from build123d import *

# Parameters (mm, degrees)
F0_W     = 150
F0_H     = 75
F1_DEPTH = 4.8
F2_W     = 143
F2_H     = 1.4
F3_DEPTH = 2
F4_R     = 1.99999


# Not quite as in the source:
# - a fillet or chamfer is up to 0.001 mm smaller than in the source, because OpenCascade refuses the exact size


with BuildPart() as f1:
    # F0 (on Front) → F1 (new body)
    with BuildSketch(Plane.XZ):
        Rectangle(F0_W, F0_H)
    extrude(amount=F1_DEPTH)

    # F2 (on face) → F3 (cut)
    with BuildSketch(Plane.XZ.offset(4.8)):
        Polygon((68, 12.5), (68, -37.5), (73, -37.5), (73, 37.5), (68, 37.5), (68, 13.9), align=None)
        with Locations((-3.5, 13.2)):
            Rectangle(F2_W, F2_H)
    extrude(amount=-F3_DEPTH, mode=Mode.SUBTRACT)

    # F4 (radius 2 in the source; OpenCascade refuses exactly that, so slightly less here)
    f4_edges = [f1.edges().sort_by_distance(p)[0] for p in [
        (75, 0, 0),
        (75, -4.8, 0),
    ]]
    fillet(f4_edges, radius=F4_R)


solid = f1.part
Geometry: final body of the model. Coordinates: model frame, mm. Coordinates: 2 decimals unless noted, no trailing zeros. Order: outer loops, then holes, each group sorted by start corner. A loop starts at its lowest first (then second) coordinate and runs counter-clockwise, first axis right, second up.
(1) First-contact query: pin 1 (2 mm diameter, centred on y = -4.5, z = -17.5, fed in from +X). Flat tip, straight axial feed; report the tip coordinate or a pass-through.
(2) Draft query along Z for faces 1 (the face through (-75, -2, -1)), 2 (the face through (-1, -2, -37.5)), 3 (the face through (-1, -2, 37.5)). Return one class per face: pulls with the +Z half, pulls with the -Z half, needs draft (parallel to the pull), parting line crosses it, or undercut.
(3) Material intervals for probe 1 along X at (y, z) = (-2.9, 3.5); probe 2 along Z at (x, y) = (41, -2.9); probe 3 along X at (y, z) = (-3.5, 34), sorted ascending.
(4) Section query B-B (y = -3.9). Return the cut outline in (x, z).
Solution:
1. pin 1: stops at x = 74.87
2. face 1: needs draft
2. face 2: pulls with the -Z half
2. face 3: pulls with the +Z half
3. probe 1: x = -75 to 68, 73 to 75
3. probe 2: z = -37.5 to 12.5, 13.9 to 37.5
3. probe 3: x = -75 to 68, 73 to 74.87
4. outline: (-75, -37.5) - (68, -37.5) - (68, 12.5) - (-75, 12.5) - close; (-75, 13.9) - (68, 13.9) - (68, 37.5) - (-75, 37.5) - close; (73, -37.5) - (74.67, -37.5) - (74.67, 37.5) - (73, 37.5) - close
